The listing builds one solid part. Answer for the finished solid, in the listing's coordinates (mm). Round coordinates to 2 decimals unless told otherwise and drop trailing zeros. Order: outer loops, then holes, each group sorted by start corner. A loop starts at its lowest first (then second) coordinate and runs counter-clockwise, first axis right, second up. Notation, with made-up numbers: (-15.5, -39) -> (-0.5, -39) arc R28 cw to (-0.5, -9) -> close; hole circle Ø2 at (-3, 73.5). An arc over 180 degrees is marked (long way). Answer in a Markdown table with one row per item. Add a question column.
```python
from build123d import *

# Parameters (mm, degrees)
BOSS_EXTRUDE1_DEPTH = 2
SKETCH2_R           = 1.5
CUT_EXTRUDE1_DEPTH  = 5.444097209
FILLET1_R           = 0.5
FILLET2_R           = 0.2
CHAMFER1_SIZE       = 0.1


with BuildPart() as part:
    # Sketch1 → Boss-Extrude1 (new body)
    with BuildSketch(Plane(origin=(0, 0, 0), x_dir=(1, 0, 0), z_dir=(0, 1, 0))):
        Polygon((3, 0), (1.5, 2.598076211), (-1.5, 2.598076211), (-3, 0), (-1.5, -2.598076211), (1.5, -2.598076211), align=None)
    extrude(amount=BOSS_EXTRUDE1_DEPTH)

    # Sketch2 → Cut-Extrude1 (cut, through all)
    with BuildSketch(Plane(origin=(0, 2, 0), x_dir=(1, 0, 0), z_dir=(0, 1, 0))):
        with Locations(Location((0, 0, 0), (0, 0, 270))):
            Circle(SKETCH2_R)
    extrude(amount=-CUT_EXTRUDE1_DEPTH, mode=Mode.SUBTRACT)

    # Fillet1
    fillet1_edges = [part.edges().sort_by_distance(p)[0] for p in [
        (1.5, 1, 2.598076211),
        (-1.5, 1, 2.598076211),
        (-3, 1, 0),
        (-1.5, 1, -2.598076211),
        (1.5, 1, -2.598076211),
        (3, 1, 0),
    ]]
    fillet(fillet1_edges, radius=FILLET1_R)

    # Fillet2
    fillet2_edges = [part.edges().sort_by_distance(p)[0] for p in [
        (0, 0, 2.598076211),
        (0, 2, 2.598076211),
        (2.25, 0, 1.299038106),
        (-2.25, 0, 1.299038106),
        (-2.25, 0, -1.299038106),
        (0, 0, -2.598076211),
        (2.25, 0, -1.299038106),
        (1.461324865, 0, 2.531088913),
        (2.922649731, 0, 0),
        (1.461324865, 0, -2.531088913),
        (-1.461324865, 0, -2.531088913),
        (-2.922649731, 0, 0),
        (-1.461324865, 0, 2.531088913),
        (-2.25, 2, 1.299038106),
        (2.25, 2, 1.299038106),
        (2.25, 2, -1.299038106),
        (0, 2, -2.598076211),
        (-2.25, 2, -1.299038106),
        (1.461324865, 2, 2.531088913),
        (2.922649731, 2, 0),
        (1.461324865, 2, -2.531088913),
        (-1.461324865, 2, -2.531088913),
        (-2.922649731, 2, 0),
        (-1.461324865, 2, 2.531088913),
    ]]
    fillet(fillet2_edges, radius=FILLET2_R)

    # Chamfer1
    chamfer1_edges = [part.edges().sort_by_distance(p)[0] for p in [
        (0, 2, -1.5),
    ]]
    chamfer(chamfer1_edges, length=CHAMFER1_SIZE)


solid = part.part
```
1. The part is cut by section C-C (x = 0). Give the vertices of the cut face in (y, z).
2. The mould has two halves that part along X. Classify faces 1 (the cylindrical face through (-2.21, 1.94, -1.25)), 2 (the cylindrical face through (0.45, 0.96, 1.43)), 3 (the cylindrical face through (2.21, 0.06, 1.25)), 4 (the flat face through (0, 0, 2)): released by +X, released by -X, zero draft, split by the parting line, or undercut.
3. The part is cut by section A-A (z = 0). Give the vertices of the cut face in (x, y).
4. This flat-tipped pin is pushed along its axis until it touches: pin 1 (3 mm diameter, centred on x = -1, z = -0.5, fed in from +Y). Where does it stop, or does it pass through?
5. The part is cut by section B-B (y = 0.35). Give the vertices of the cut face in (x, z), then the cut area to 3 significant figures.
6. Straight lines are drawn through the part: line 1 along X through (y, z) = (0.7, 0); line 2 along Z through (x, y) = (0.95, 1); line 3 along Z through (x, y) = (-1.2, 1). For each, find the intervals that lie inside material, in ascending order.
Report:
| question | item | result |
|---|---|---|
| 1 | outline | (0, -2.4) arc R0.2 ccw to (0.2, -2.6) -> (1.8, -2.6) arc R0.2 ccw to (2, -2.4) -> (2, -1.6) -> (1.9, -1.5) -> (0, -1.5) -> close; (0, 1.5) -> (1.9, 1.5) -> (2, 1.6) -> (2, 2.4) arc R0.2 ccw to (1.8, 2.6) -> (0.2, 2.6) arc R0.2 ccw to (0, 2.4) -> close |
| 2 | face 1 | released by -X |
| 2 | face 2 | undercut |
| 2 | face 3 | released by +X |
| 2 | face 4 | zero draft |
| 3 | outline | (-2.92, 0.2) arc R0.2 ccw to (-2.72, 0) -> (-1.5, 0) -> (-1.5, 1.9) -> (-1.6, 2) -> (-2.72, 2) arc R0.2 ccw to (-2.92, 1.8) -> close; (1.5, 0) -> (2.72, 0) arc R0.2 ccw to (2.92, 0.2) -> (2.92, 1.8) arc R0.2 ccw to (2.72, 2) -> (1.6, 2) -> (1.5, 1.9) -> close |
| 4 | pin 1 | stops at y = 2 |
| 5 | outline | (-2.86, -0.25) -> (-1.64, -2.35) arc R0.5 ccw to (-1.21, -2.6) -> (1.21, -2.6) arc R0.5 ccw to (1.64, -2.35) -> (2.86, -0.25) arc R0.5 ccw to (2.86, 0.25) -> (1.64, 2.35) arc R0.5 ccw to (1.21, 2.6) -> (-1.21, 2.6) arc R0.5 ccw to (-1.64, 2.35) -> (-2.86, 0.25) arc R0.5 ccw to start; hole circle Ø3 at (0, 0) |
| 5 | area | 16.2 mm^2 |
| 6 | line 1 | x = -2.92 to -1.5, 1.5 to 2.92 |
| 6 | line 2 | z = -2.6 to -1.16, 1.16 to 2.6 |
| 6 | line 3 | z = -2.6 to -0.9, 0.9 to 2.6 |
